Source: three-view drawing plus pictorial views. Frame: mm from the lowest corner of the part. A direction names the side the tool comes from. Round coordinates to 2 decimals unless told otherwise and drop trailing zeros. Loops run counter-clockwise (first coordinate to the right, second up) from the corner with the lowest first, then second, coordinate; pieces in that order, holes last. Notation, with made-up numbers: M -9.75,16 L 33.25,16 A10 cw 33.25,23 Z; hole C 25,62 d1. An arc over 180 degrees is marked long. Answer as a JSON object with one key per item and string values.
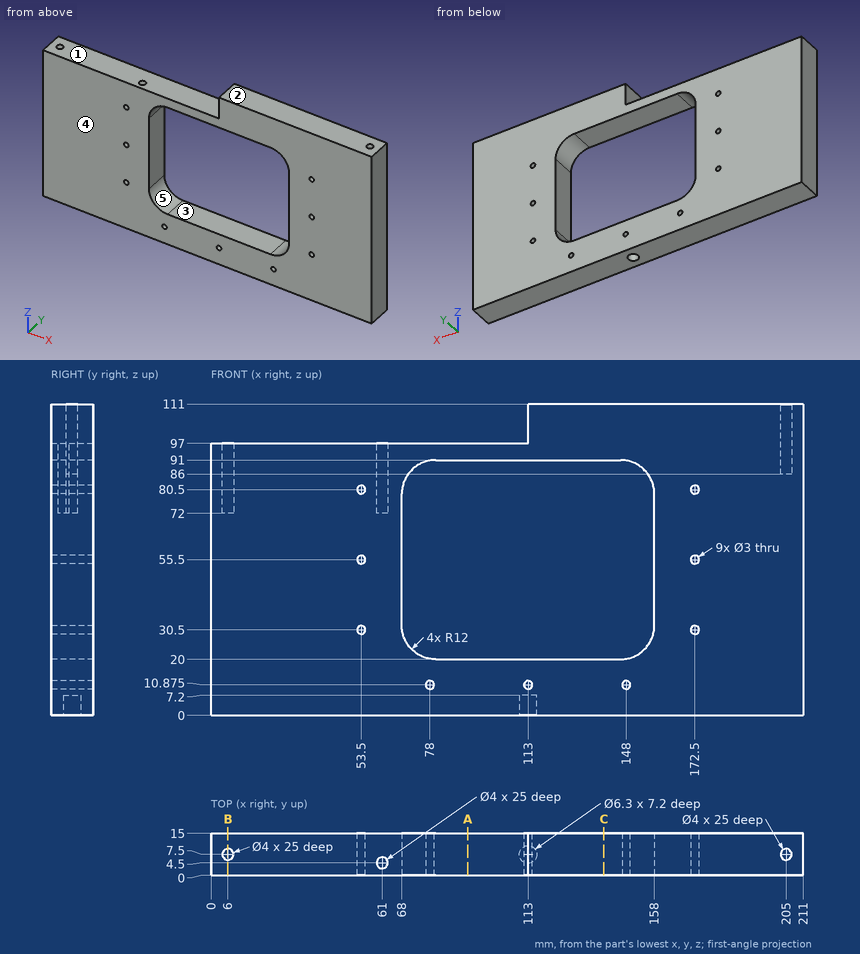
1) Cut plane B-B on x = 6. Return the cut outline in (y, z).
Geometry results:
{"outline": "M 0,0 L 15,0 L 15,97 L 9.5,97 L 9.5,72 L 5.5,72 L 5.5,97 L 0,97 Z"}
2) Pull-direction query (X, two-part tool) for the marked faces 4 and 5; classes: +X half, -X half, draft (parallel to the pull), parting line (faces both ways), or undercut.
Geometry results:
{"face 4": "draft", "face 5": "undercut"}
3) Line query: probe 1 along Z at (x, y) = (53.5, 8); probe 2 along Z at (x, y) = (138.5, 11.5); probe 3 along Y at (x, z) = (205, 99.25). Output: solid intervals per line, ascending.
Geometry results:
{"probe 1": "0 to 29, 32 to 54, 57 to 79, 82 to 97", "probe 2": "0 to 20, 91 to 111", "probe 3": "0 to 5.5, 9.5 to 15"}
4) Set-up query: the marked faces 1, 2 and 3. Return all of +Z, -Z, +X, -X, +Y, -Y with unobstructed straight access to the full face (end or side cutting, diameter ignored); none if empty.
Geometry results:
{"face 1": "+Z, -X, +Y, -Y", "face 2": "+Z, +X, -X, +Y, -Y", "face 3": "+Y, -Y"}
5) Cut plane A-A on x = 91.5. Return the cut outline in (y, z), and give its area (3 significant figures).
Geometry results:
{"outline": "M 0,0 L 15,0 L 15,20 L 0,20 Z; M 0,91 L 15,91 L 15,97 L 0,97 Z", "area": "390 mm2"}
6) Cut plane C-C on x = 140. Return the cut outline in (y, z).
Geometry results:
{"outline": "M 0,0 L 15,0 L 15,20 L 0,20 Z; M 0,91 L 15,91 L 15,111 L 0,111 Z"}
7) First-contact query: pin 1 (1.2 mm diameter, centred on x = 204.5, y = 8, fed in from +Z); pin 2 (3 mm diameter, centred on x = 114, y = 7.5, fed in from -Z); pin 3 (1 mm diameter, centred on x = 30, y = 6.5, fed in from +Z). Flat tips, straight axial feed; report the tip coordinate or a pass-through.
Geometry results:
{"pin 1": "z = 86", "pin 2": "z = 7.2", "pin 3": "z = 97"}
